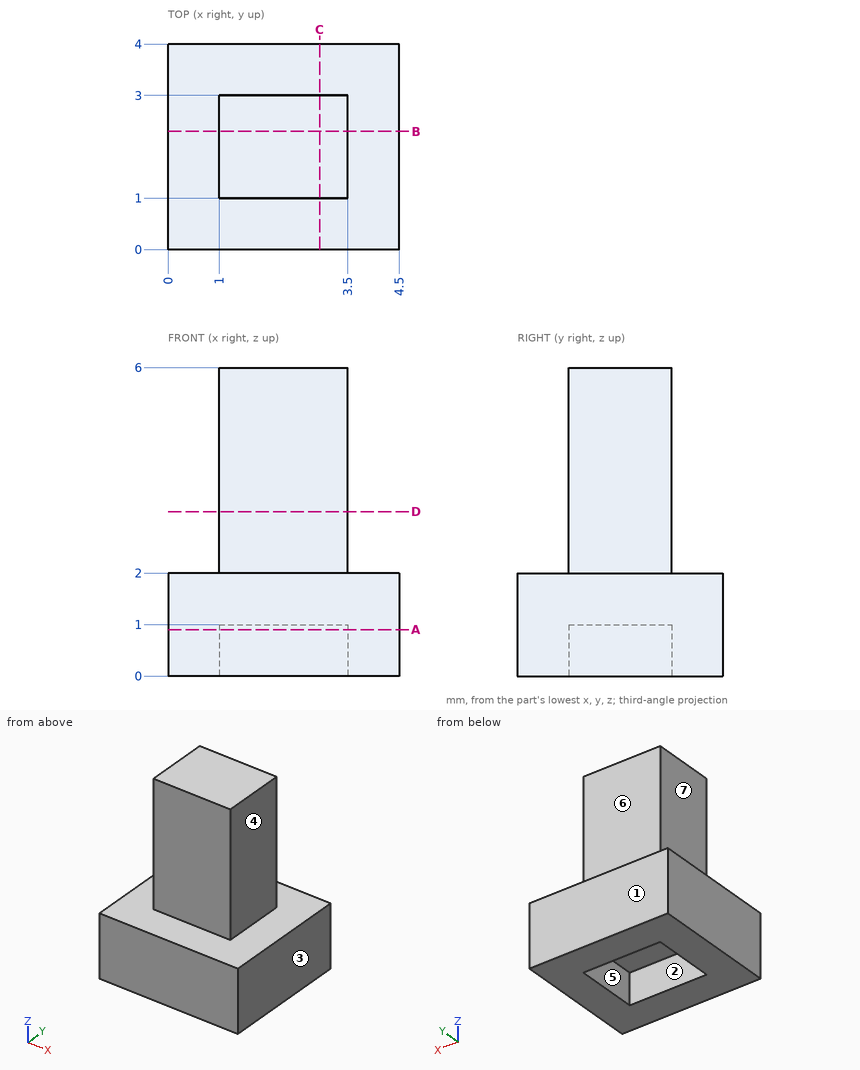
Geometry check sheet. Reference: drawing and pictorial views, mm from the part's lowest x, y, z. A direction names the side the tool comes from. Round coordinates to 2 decimals unless told otherwise and drop trailing zeros. Loops run counter-clockwise (first coordinate to the right, second up) from the corner with the lowest first, then second, coordinate; pieces in that order, holes last.
1. Sectioned sample at D-D on z = 3.2. Record the boundary of the cut face in (x, y).
2. Sectioned sample at C-C on x = 2.95. Record the boundary of the cut face in (y, z), and give its area (3 significant figures).
3. Sectioned sample at A-A on z = 0.9. Record the boundary of the cut face in (x, y).
4. Scan lines: probe 1 along X at (y, z) = (2.4, 2.75); probe 2 along Z at (x, y) = (2.55, 0.3); probe 3 along Z at (x, y) = (2.75, 2.9). Record each from-to range of solid material in increasing order.
5. Sectioned sample at B-B on y = 2.3. Record the boundary of the cut face in (x, z), and give its area (3 significant figures).
6. Gauge pin test, flat ends, axial feed: pin 1 Ø0.6 at (y, z) = (2, 4) entering from -X; pin 2 Ø2 at (y, z) = (2, 4.5) entering from +X; pin 3 Ø1.5 at (x, z) = (4, 5.5) entering from +Y. Record the tip position at first contact, or that the pin passes through.
7. Set-up check for the marked faces 4, 5, 6 and 7: record each of +Z, -Z, +X, -X, +Y, -Y from which the full face is reachable in a straight line by a thin tool's end or side.
8. Mould release check, pull along X, two halves, no side actions. Record for the marked faces 1, 2 and 3: released by +X, released by -X, zero draft, split by the parting line, or undercut.
Recorded:
1. outline: (1, 1) - (3.5, 1) - (3.5, 3) - (1, 3) - close
2. outline: (0, 0) - (1, 0) - (1, 1) - (3, 1) - (3, 0) - (4, 0) - (4, 2) - (3, 2) - (3, 6) - (1, 6) - (1, 2) - (0, 2) - close
2. area: 14.0 mm2
3. outline: (0, 0) - (4.5, 0) - (4.5, 4) - (0, 4) - close; hole (1, 1) - (3.5, 1) - (3.5, 3) - (1, 3) - close
4. probe 1: x = 1 to 3.5
4. probe 2: z = 0 to 2
4. probe 3: z = 1 to 6
5. outline: (0, 0) - (1, 0) - (1, 1) - (3.5, 1) - (3.5, 0) - (4.5, 0) - (4.5, 2) - (3.5, 2) - (3.5, 6) - (1, 6) - (1, 2) - (0, 2) - close
5. area: 16.5 mm2
6. pin 1: stops at x = 1
6. pin 2: stops at x = 3.5
6. pin 3: stops at y = 3
7. face 4: +Z, +X, +Y, -Y
7. face 5: -Z
7. face 6: +Z, +X, -X, +Y
7. face 7: +Z, -X, +Y, -Y
8. face 1: zero draft
8. face 2: undercut
8. face 3: released by +X
